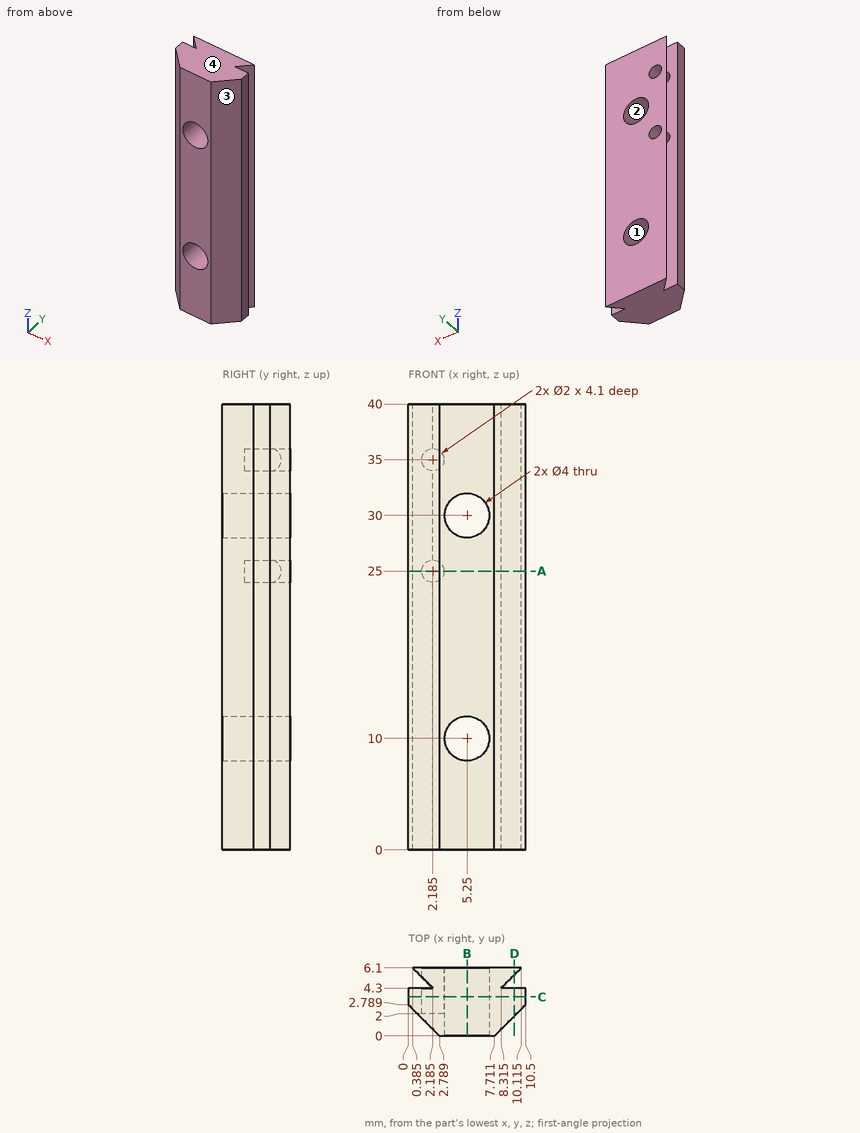
Geometry: see drawing. Coordinates: mm, zero at the bounding-box minimum. Give positions to 0.01 mm unless a question says otherwise; leave off trailing zeros. Loops run counter-clockwise (first coordinate to the right, second up) from the corner with the lowest first, then second, coordinate; pieces in that order, holes last. Notation, with made-up numbers: M 56.25,7 L 76.25,7 A34 ccw 76.25,43 Z; hole C -31.75,89 d11. An arc over 180 degrees is marked long. Answer as CSV lines item,"result". Start each with the question number.
1. Section B-B on x = 5.25. Return loops of the section in (y, z).
2. Line query: L1, parallel to Z at x = 5.25, y = 2.5; L2, parallel to X at y = 3.75, z = 35 (1 decimal); L3, parallel to Z at x = 1.5, y = 3.75. Output: solid intervals per line, ascending.
3. Pull-direction query (X, two-part tool) for the marked faces 1, 2, 3 and 4; classes: released by +X, released by -X, zero draft, split by the parting line, or undercut.
4. Section A-A on z = 25. Return loops of the section in (x, y) (1 decimal).
5. Section D-D on x = 9.5. Return loops of the section in (y, z) (1 decimal), plus the area to 3 significant figures.
6. Section C-C on y = 3.5. State how many separate pieces and enclosed holes the cut face has.
Computed values:
1,outline,"M 0,0 L 6.1,0 L 6.1,8 L 0,8 Z; M 0,12 L 6.1,12 L 6.1,28 L 0,28 Z; M 0,32 L 6.1,32 L 6.1,40 L 0,40 Z"
2,L1,"z = 0 to 8, 12 to 28, 32 to 40"
2,L2,"x = 0 to 1.2, 3.2 to 10.5"
2,L3,"z = 0 to 24.27, 25.73 to 34.27, 35.73 to 40"
3,face 1,"undercut"
3,face 2,"undercut"
3,face 3,"released by +X"
3,face 4,"zero draft"
4,outline,"M 0,2.8 L 2.8,0 L 7.7,0 L 10.5,2.8 L 10.5,4.3 L 8.3,4.3 L 10.1,6.1 L 3.2,6.1 L 3.2,2 L 1.2,2 L 1.2,4.3 L 0,4.3 Z; M 0.4,6.1 L 1.2,5.3 L 1.2,6.1 Z"
5,outline,"M 1.8,0 L 4.3,0 L 4.3,40 L 1.8,40 Z; M 5.5,0 L 6.1,0 L 6.1,40 L 5.5,40 Z"
5,area,"125 mm²"
6,separate pieces,"1"
6,enclosed holes,"4"
